For this review, use the dimensioned drawing (mm, ordinates from the lowest corner) and the shaded views. Coordinates: 2 decimals unless noted, no trailing zeros. Write each loop counter-clockwise with the first axis right and the second up, starting at its lowest first coordinate (ties: lowest second). Pieces come first, ordered by that corner, then holes. Notation, with made-up numbers: (-31, 47) - (-10, 47) arc R23 ccw to (-10, 68) - close; hole circle Ø2 at (32, 27.25). An arc over 180 degrees is marked (long way). Put each result on its own line as item: value.
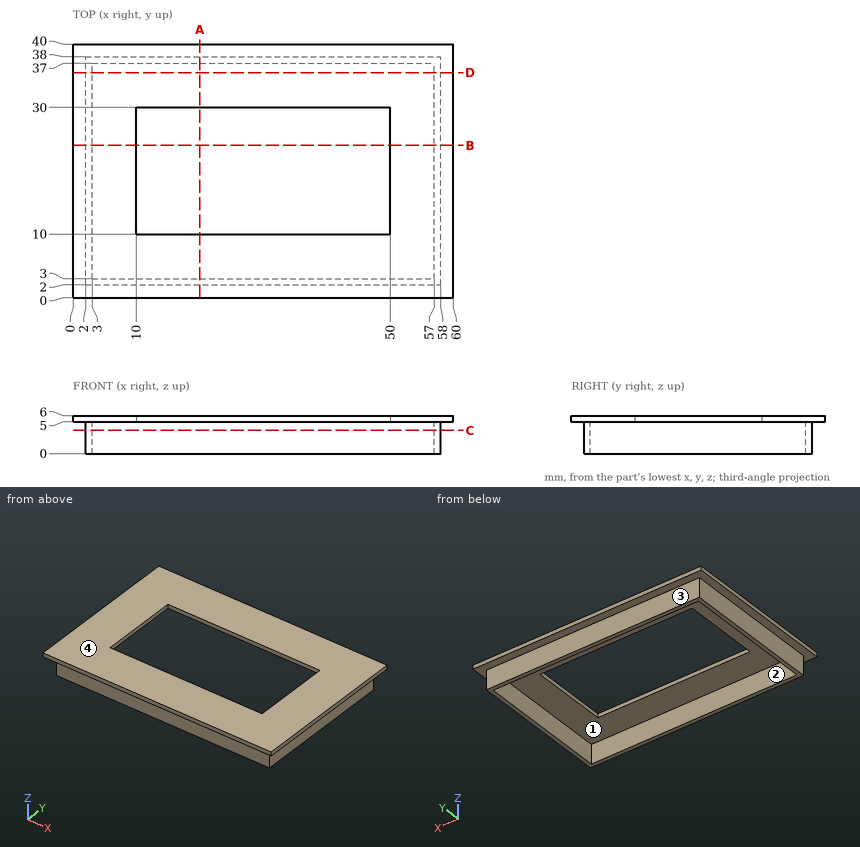
1. Consider section C-C on z = 3.65. State the section outline as (x, y) points, plus the area to 3 significant figures.
Determined:
outline: (2, 2) - (58, 2) - (58, 38) - (2, 38) - close; hole (3, 3) - (57, 3) - (57, 37) - (3, 37) - close
area: 180 mm^2
2. Consider section B-B on y = 24. State the section outline as (x, z) points.
Determined:
outline: (0, 5) - (2, 5) - (2, 0) - (3, 0) - (3, 5) - (10, 5) - (10, 6) - (0, 6) - close; (50, 5) - (57, 5) - (57, 0) - (58, 0) - (58, 5) - (60, 5) - (60, 6) - (50, 6) - close
3. To check wall thickness, follow probe 1 along X at (y, z) = (16.5, 0.7); probe 2 along Y at (x, z) = (48.5, 0.75); probe 3 along Y at (x, z) = (27, 5.65). State the ranges of each line that lie inside material, in increasing order.
Determined:
probe 1: x = 2 to 3, 57 to 58
probe 2: y = 2 to 3, 37 to 38
probe 3: y = 0 to 10, 30 to 40
4. Consider section A-A on x = 20. State the section outline as (y, z) points.
Determined:
outline: (0, 5) - (2, 5) - (2, 0) - (3, 0) - (3, 5) - (10, 5) - (10, 6) - (0, 6) - close; (30, 5) - (37, 5) - (37, 0) - (38, 0) - (38, 5) - (40, 5) - (40, 6) - (30, 6) - close
5. For pin 1 Ø1.1 at (x, z) = (35, 5.5) entering from -Y; pin 2 Ø4 at (x, y) = (13.5, 27) entering from +Z; pin 3 Ø1.5 at (y, z) = (19.5, 2.5) entering from -X; pin 4 Ø2.5 at (x, z) = (29, 2.5) entering from -Y, all flat-tipped, find the tip position at first contact; note any pin that passes through.
Determined:
pin 1: stops at y = 0
pin 2: passes through
pin 3: stops at x = 2
pin 4: stops at y = 2
6. Consider section D-D on y = 35.5. State the section outline as (x, z) points.
Determined:
outline: (0, 5) - (2, 5) - (2, 0) - (3, 0) - (3, 5) - (57, 5) - (57, 0) - (58, 0) - (58, 5) - (60, 5) - (60, 6) - (0, 6) - close
7. The part is to be moulded in two halves that separate along Y. For the marked faces 1, 2, 3 and 4, say which applies: +Y half, -Y half, draft (parallel to the pull), parting line (faces both ways), or undercut.
Determined:
face 1: undercut
face 2: undercut
face 3: +Y half
face 4: draft
